Here's the drawing with two shaded views (mm, measured from the low corner). I have some questions. A direction names the side the tool comes from. Coordinates: 2 decimals unless noted, no trailing zeros. Loops run counter-clockwise (first coordinate to the right, second up) from the corner with the lowest first, then second, coordinate; pieces in that order, holes last. Notation, with made-up numbers: M 37.5,59 L 59.5,59 A4 cw 59.5,66 Z; hole C 30,75 d7. An arc over 180 degrees is marked long. Return JSON: item names as keys, results as strings. Group by question number.
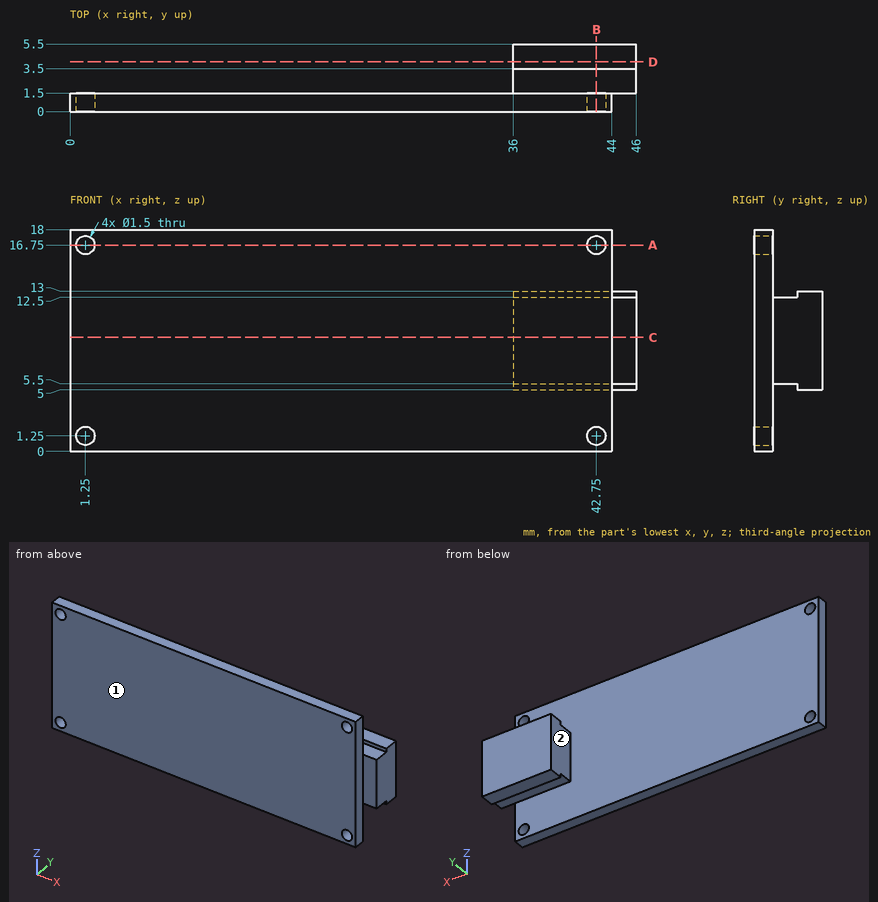
1) Suppose I cut it at C-C, the plane z = 9.25. List the corners of the cut face in (x, y) for me, then the cut area to 3 significant figures.
2) Suppose I cut it at D-D, the plane y = 4.05. List the corners of the cut face in (x, z) for me, then the cut area to 3 significant figures.
3) For the marked faces 1 and 2, which set-ups out of +Z, -Z, +X, -X, +Y, -Y let a thin tool reach every point of the face, with its end or its side?
4) Suppose I cut it at B-B, the plane x = 42.75. List the corners of the cut face in (y, z) for me, then the cut area to 3 significant figures.
5) If I drill on line 1 (Z direction, x = 42.75, y = 1.1); line 2 (X direction, y = 0.3, z = 1.25); line 3 (X direction, y = 3.05, z = 11.75), over which ranges is the centre line in solid material (lowest first)? Write a range as from..to.
6) Suppose I cut it at A-A, the plane z = 16.75. List the corners of the cut face in (x, y) for me, then the cut area to 3 significant figures.
7) For pin 1 (2 mm diameter, centred on x = 44.5, z = 8.5, fed in from -Y); pin 2 (0.9 mm diameter, centred on x = 42.75, z = 16.75, fed in from -Y); pin 3 (0.6 mm diameter, centred on x = 39, y = 4.5, fed in from -Z); pin 4 (1.7 mm diameter, centred on x = 1.25, z = 1.25, fed in from +Y), each with a flat end and sliding along its axis, tell me the tip position at first contact or that it passes through.
Returned:
{
 "1": {"outline": "M 0,0 L 44,0 L 44,1.5 L 46,1.5 L 46,5.5 L 36,5.5 L 36,1.5 L 0,1.5 Z", "area": "106 mm²"},
 "2": {"outline": "M 36,5 L 46,5 L 46,13 L 36,13 Z", "area": "80.0 mm²"},
 "3": {"face 1": "+Z, -Z, +X, -X, -Y", "face 2": "+Z, -Z, -X, +Y"},
 "4": {"outline": "M 0,0 L 1.5,0 L 1.5,0.5 L 0,0.5 Z; M 0,2 L 1.5,2 L 1.5,5.5 L 3.5,5.5 L 3.5,5 L 5.5,5 L 5.5,13 L 3.5,13 L 3.5,12.5 L 1.5,12.5 L 1.5,16 L 0,16 Z; M 0,17.5 L 1.5,17.5 L 1.5,18 L 0,18 Z", "area": "52.5 mm²"},
 "5": {"line 1": "z = 0..0.5, 2..16, 17.5..18", "line 2": "x = 0..0.5, 2..42, 43.5..44", "line 3": "x = 36..46"},
 "6": {"outline": "M 0,0 L 0.5,0 L 0.5,1.5 L 0,1.5 Z; M 2,0 L 42,0 L 42,1.5 L 2,1.5 Z; M 43.5,0 L 44,0 L 44,1.5 L 43.5,1.5 Z", "area": "61.5 mm²"},
 "7": {"pin 1": "stops at y = 0", "pin 2": "passes through", "pin 3": "stops at z = 5", "pin 4": "stops at y = 1.5"}
}
